Autodesk Inventor part; units mm, degrees
ref_plane "YZ Plane" through (0, 0, 0) normal (1, 0, 0) x (0, 1, 0)
ref_plane "XZ Plane" through (0, 0, 0) normal (0, 1, 0) x (-1, 0, 0)
ref_plane "XY Plane" through (0, 0, 0) normal (0, 0, 1) x (1, 0, 0)
sketch "Sketch1" plane through (0, 0, 0) normal (0, 0, 1) x (1, 0, 0)
  line L0 (6.35, -22.225) -> (-6.35, -22.225)
  line L1 (-6.35, -22.225) -> (-6.35, 22.225)
  line L2 (-6.35, 22.225) -> (6.35, 22.225)
  line L3 (6.35, 22.225) -> (6.35, -22.225)
  line L4 (6.35, -22.225) -> (-6.35, 22.225) construction
  line L5 (-6.35, -22.225) -> (6.35, 22.225) construction
  point P0 (0, 0)
  dimension "d0" = 12.7
  dimension "d6" = 44.45
extrude "Plate1" add sketch "Sketch1" along normal blind 12.7
sketch "Sketch2" plane through (6.35, -22.225, 0) normal (1, 0, 0) x (0, 0, -1)
  line L0 (0, 0) -> (-12.7, 0)
  line L1 (0, 0) -> (0, 44.45)
  point P0 (0, 22.225)
  point P1 (-6.35, 6.35)
  point P2 (-6.35, 19.05)
  point P3 (-6.35, 31.75)
  dimension "d2" = 6.35
  dimension "d3" = 12.7
  dimension "d4" = 12.7
  dimension "d5" = 6.35
hole "Hole1" at (6.35, -15.875, 6.35) at (6.35, -3.175, 6.35) at (6.35, 9.525, 6.35) direction (-1, 0, 0) diameter 3.9624 depth 12.7 tip angle 118
sketch "Sketch3" plane through (0, 0, 12.7) normal (0, 0, 1) x (1, 0, 0)
  line L0 (-6.35, 22.225) -> (6.35, 22.225)
  point P0 (0, 0)
  point P1 (0, -9.525)
  point P2 (0, 3.175)
  point P3 (0, 15.875)
  dimension "d14" = 12.7
  dimension "d15" = 12.7
  dimension "d16" = 6.35
hole "Hole2" at (0, -9.525, 12.7) at (0, 3.175, 12.7) at (0, 15.875, 12.7) direction (0, 0, -1) diameter 3.9624 depth 12.7 tip angle 118
fillet "Corner Round1" radius 1.5875 4 edges at (6.35, -22.225, 6.35) (-6.35, -22.225, 6.35) (6.35, 22.225, 6.35) (-6.35, 22.225, 6.35)
equation "\"d22\" = Thickness"
equation "\"d1\" = Thickness"
equation "\"BendRadius\" = Thickness"
equation "\"BendReliefWidth\" = Thickness"
equation "\"BendReliefDepth\" = 0.5 * Thickness"
equation "\"CornerReliefSize\" = 4 * Thickness"
equation "\"MinimumRemnant\" = 2 * Thickness"
equation "\"TransitionRadius\" = BendRadius"
equation "\"JacobiRadiusSize\" = BendRadius"
equation "\"GapSize\" = Thickness"
properties part number "PLATE,NUT-BLOCK,3-LONG" material "Aluminum 6061"
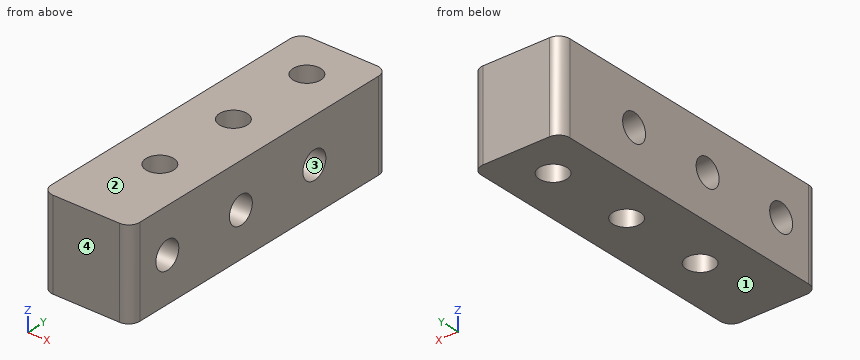
Check sheet for the modelled part. Datum: model origin and axes. Units: mm. Face numbers are marked on the shaded views. Round coordinates to 2 decimals unless told otherwise and drop trailing zeros. Loops run counter-clockwise (first coordinate to the right, second up) from the corner with the lowest first, then second, coordinate; pieces in that order, holes last. Notation, with made-up numbers: (52, 1.25) -> (82, 1.25) arc R34 ccw to (82, 32.25) -> close; hole circle Ø5 at (56.5, 62.5). An arc over 180 degrees is marked (long way). Put each result on its own line as item: value. Start each with the question number.
1. Gauge pin test, flat end, axial feed: pin 1 (5 mm diameter, centred on x = 0, y = 3.175, fed in from -Z). Record the tip position at first contact, or that the pin passes through.
2. Section check A-A (z = 6.35). Give the number of separate pieces and of enclosed holes in the cut face, plus the area to 3 significant figures.
3. Section check B-B (x = -1). Enter the section's corners in (y, z) (3 decimals), plus the area to 3 significant figures.
4. Scan lines: probe 1 along Y at (x, z) = (2.5, 6.35) (3 decimals); probe 2 along Y at (x, z) = (-1.5, 3.5) (3 decimals); probe 3 along Z at (x, y) = (2, -16). Record each from-to range of solid material in increasing order.
5. Section check C-C (y = 4.5). Enter the section's corners in (x, z), plus the area to 3 significant figures.
6. Draft check along Z on the marked faces 1, 2, 3 and 4. Enter one of: +Z half, -Z half, draft (parallel to the pull), parting line (faces both ways), or undercut.
Findings:
1. pin 1: stops at z = 0
2. separate pieces: 4
2. enclosed holes: 3
2. area: 374 mm^2
3. outline: (-22.225, 0) -> (-11.235, 0) -> (-11.235, 12.7) -> (-22.225, 12.7) -> close; (-7.815, 0) -> (1.465, 0) -> (1.465, 12.7) -> (-7.815, 12.7) -> close; (4.885, 0) -> (14.165, 0) -> (14.165, 12.7) -> (4.885, 12.7) -> close; (17.585, 0) -> (22.225, 0) -> (22.225, 12.7) -> (17.585, 12.7) -> close; hole circle Ø3.962 at (-15.875, 6.35); hole circle Ø3.962 at (-3.175, 6.35); hole circle Ø3.962 at (9.525, 6.35)
3. area: 397 mm^2
4. probe 1: y = -22.225 to -17.856, -13.894 to -5.156, -1.194 to 7.544, 11.506 to 22.225
4. probe 2: y = -22.225 to -10.819, -8.231 to 1.881, 4.469 to 14.581, 17.169 to 22.225
4. probe 3: z = 0 to 4.37, 8.33 to 12.7
5. outline: (-6.35, 0) -> (-1.47, 0) -> (-1.47, 12.7) -> (-6.35, 12.7) -> close; (1.47, 0) -> (6.35, 0) -> (6.35, 12.7) -> (1.47, 12.7) -> close
5. area: 124 mm^2
6. face 1: -Z half
6. face 2: +Z half
6. face 3: undercut
6. face 4: draft
